For this review, take the finished solid that the model builds, in its own axes (mm). A direction names the side the tool comes from. Give positions to 0.01 mm unless a question says otherwise; leave off trailing zeros. Order: outer loops, then holes, each group sorted by start corner. A loop starts at its lowest first (then second) coordinate and runs counter-clockwise, first axis right, second up. Notation, with made-up numbers: (55, 50.5) -> (85, 50.5) arc R33 cw to (85, 86.5) -> close; hole circle Ø2 at (-9, 5). An arc over 180 degrees is marked (long way). Return JSON: item names as keys, results as strings. Group by question number.
1) Add section B-B (x = -17.8). Give the boundary of the cut face in (y, z), then the cut area to 4 significant figures.
2) Add section A-A (z = 15.5). Give the boundary of the cut face in (x, y), then the cut area to 3 significant figures.
3) Insertion check: P1, Ø2, axis at x = -17.8, z = 15.5, coming from the -Y side; P2, Ø7.5, axis at y = -9.5, z = 3, coming from the +X side; P3, Ø1.5, axis at y = -4.5, z = 9, coming from the +X side; P4, Ø8, axis at x = 10.5, y = -19.5, coming from the -Z side. Each pin has a flat end and moves straight along its axis. Give the tip position at first contact, or say it passes through.
4) For faces 1 (the face through (11.91, -15.62, 16.68)), 2 (the face through (16, -3.5, 23)), 3 (the face through (-1.05, -19, -15)), 4 (the face through (-16.9, -12.3, -14)), list the 3-axis set-ups (+Z, -Z, +X, -X, +Y, -Y) from which the entire face can be reached by the end or side of a thin tool; tool diameter is ignored.
5) Add section D-D (x = -2.3). Give the boundary of the cut face in (y, z), then the cut area to 4 significant figures.
6) To check wall thickness, follow line 1 along Z through (x, y) = (-17.8, -11.25); line 2 along X through (y, z) = (-16.25, 0); line 3 along X through (y, z) = (-19.5, -11). State the ranges of each line that lie inside material, in increasing order.
7) Add section C-C (y = -17.25). Give the boundary of the cut face in (x, z), then the cut area to 3 significant figures.
8) The part is to be moulded in two halves that separate along Z. For faces 5 (the face through (13, -3.5, 16)), 6 (the face through (16, -6.5, 23)), 7 (the face through (-21.4, -12.3, 19.2)), 8 (the face through (14.869, -4.774, -14.974)), say which applies: released by +Z, released by -Z, zero draft, split by the parting line, or undercut.
from build123d import *

# Parameters (mm, degrees)
F0_W      = 46.9
F0_H      = 42.3
F0_R      = 1.75
F1_DEPTH  = 25
F2_SIZE   = 4
F4_DEPTH  = 12.7
F5_R      = 2.1
F6_DEPTH  = 29.601
F7_SIZE   = 2
F9_DEPTH  = 25.0010001
F11_R     = 14
F12_DEPTH = 1.5


# Not quite as in the source:
# - a feature names something its author has since deleted; it is built from what else it names


with BuildPart() as f1:
    # F0 (on Front) → F1 (new body)
    with BuildSketch(Plane.XZ):
        Rectangle(F0_W, F0_H)
        with Locations((-17.8, -15.5)):
            Circle(F0_R, mode=Mode.SUBTRACT)
        with Locations((13.2, -15.5)):
            Circle(F0_R, mode=Mode.SUBTRACT)
        with Locations((-17.8, 15.5)):
            Circle(F0_R, mode=Mode.SUBTRACT)
        with Locations((13.2, 15.5)):
            Circle(F0_R, mode=Mode.SUBTRACT)
    extrude(amount=F1_DEPTH)

    # F2
    f2_edges = [f1.edges().sort_by_distance(p)[0] for p in [
        (-23.45, -12.5, 21.15),
        (23.45, -12.5, 21.15),
        (23.45, -12.5, -21.15),
        (-23.45, -12.5, -21.15),
    ]]
    chamfer(f2_edges, length=F2_SIZE)

    # F3 (on face) → F4 (cut)
    with BuildSketch(Plane(origin=(0, 0, -21.15), x_dir=(1, 0, 0), z_dir=(0, 0, -1))):
        with BuildLine():
            Line((6.95, 12.5), (14.95, 12.5))
            ThreePointArc((14.95, 12.5), (6.95, 20.5), (-1.05, 12.5))
            Line((-1.05, 12.5), (6.95, 12.5))
        make_face()
        with BuildLine():
            ThreePointArc((-1.05, 12.5), (6.95, 4.5), (14.95, 12.5))
            Line((14.95, 12.5), (6.95, 12.5))
            Line((6.95, 12.5), (-1.05, 12.5))
        make_face()
        with BuildLine():
            ThreePointArc((-1.05, 12.5), (6.95, 20.5), (14.95, 12.5))
            Line((14.95, 12.5), (14.95, 25))
            Line((14.95, 25), (-1.05, 25))
            Line((-1.05, 25), (-1.05, 12.5))
        make_face()
    extrude(amount=-F4_DEPTH, mode=Mode.SUBTRACT)

    # F5 (on face) → F6 (cut, through all)
    with BuildSketch(Plane(origin=(0, 0, -8.45), x_dir=(1, 0, 0), z_dir=(0, 0, -1))):
        with Locations((6.95, 12.5)):
            Circle(F5_R)
    extrude(amount=-F6_DEPTH, mode=Mode.SUBTRACT)

    # F7
    f7_edges = [f1.edges().sort_by_distance(p)[0] for p in [
        (4.85, -12.5, -8.45),
        (4.85, -12.5, 21.15),
    ]]
    chamfer(f7_edges, length=F7_SIZE)

    # F8 (on face) → F9 (cut, through all)
    with BuildSketch(Plane.XZ.offset(25)):
        with BuildLine():
            Line((-16.05, 15.5), (-17.8, 15.5))
            Line((-17.8, 15.5), (-16.5625631329, 14.2625631329))
            ThreePointArc((-16.5625631329, 14.2625631329), (-16.1832108181, 14.8303039934), (-16.05, 15.5))
        make_face()
        with BuildLine():
            Line((13.2, 15.5), (11.45, 15.5))
            ThreePointArc((11.45, 15.5), (11.5832108181, 14.8303039934), (11.9625631329, 14.2625631329))
            Line((11.9625631329, 14.2625631329), (13.2, 15.5))
        make_face()
        with BuildLine():
            ThreePointArc((-16.05, -15.5), (-16.1832108181, -14.8303039934), (-16.5625631329, -14.2625631329))
            Line((-16.5625631329, -14.2625631329), (-17.8, -15.5))
            Line((-17.8, -15.5), (-16.05, -15.5))
        make_face()
        with BuildLine():
            Line((3.0033008589, 5.3033008589), (-2.3, 0))
            Line((-2.3, 0), (3.0033008589, -5.3033008589))
            ThreePointArc((3.0033008589, -5.3033008589), (4.6290964938, -2.8701257427), (5.2, 0))
            ThreePointArc((5.2, 0), (4.6290964938, 2.8701257427), (3.0033008589, 5.3033008589))
        make_face()
        with BuildLine():
            ThreePointArc((3.0033008589, 5.3033008589), (-2.3, 7.5), (-7.6033008589, 5.3033008589))
            Line((-7.6033008589, 5.3033008589), (-2.3, 0))
            Line((-2.3, 0), (3.0033008589, 5.3033008589))
        make_face()
        with BuildLine():
            Line((-2.3, 0), (-7.6033008589, 5.3033008589))
            ThreePointArc((-7.6033008589, 5.3033008589), (-9.8, 0), (-7.6033008589, -5.3033008589))
            Line((-7.6033008589, -5.3033008589), (-2.3, 0))
        make_face()
        with BuildLine():
            Line((3.0033008589, -5.3033008589), (-2.3, 0))
            Line((-2.3, 0), (-7.6033008589, -5.3033008589))
            ThreePointArc((-7.6033008589, -5.3033008589), (-2.3, -7.5), (3.0033008589, -5.3033008589))
        make_face()
    extrude(amount=-F9_DEPTH, mode=Mode.SUBTRACT)

    # F11 (on offset) → F12 (join, symmetric)
    with BuildSketch(Plane.XZ.offset(5)):
        with Locations((13.2, 15.5)):
            Circle(F11_R)
    extrude(amount=F12_DEPTH, both=True)


solid = f1.part
Evaluation:
{
 "1": {"outline": "(-25, -21.15) -> (0, -21.15) -> (0, -17.25) -> (-25, -17.25) -> close; (-25, -13.75) -> (0, -13.75) -> (0, 13.75) -> (-25, 13.75) -> close; (-25, 17.25) -> (0, 17.25) -> (0, 21.15) -> (-25, 21.15) -> close", "area": "882.5 mm^2"},
 "2": {"outline": "(-23.45, -25) -> (-19.55, -25) -> (-19.55, 0) -> (-23.45, 0) -> close; (-16.05, -25) -> (11.45, -25) -> (11.45, -6.5) -> (14.95, -6.5) -> (14.95, -25) -> (23.45, -25) -> (23.45, -6.5) -> (27.2, -6.5) -> (27.2, -3.5) -> (23.45, -3.5) -> (23.45, 0) -> (14.95, 0) -> (14.95, -3.5) -> (11.45, -3.5) -> (11.45, 0) -> (-16.05, 0) -> close; hole circle Ø4.2 at (6.95, -12.5)", "area": "1,010 mm^2"},
 "3": {"P1": "through", "P2": "x = 23.45", "P3": "x = 25.96", "P4": "z = -8.45"},
 "4": {"face 1": "-Y", "face 2": "+Z, +X, +Y", "face 3": "-Z, -Y", "face 4": "+Y, -Y"},
 "5": {"outline": "(-25, -21.15) -> (0, -21.15) -> (0, -7.5) -> (-25, -7.5) -> close; (-25, 7.5) -> (0, 7.5) -> (0, 21.15) -> (-25, 21.15) -> close", "area": "682.5 mm^2"},
 "6": {"line 1": "-21.15 to -17.25, -13.75 to 13.75, 17.25 to 21.15", "line 2": "-23.45 to -9.8, 5.2 to 23.45", "line 3": "-23.45 to -1.05, 14.95 to 23.45"},
 "7": {"outline": "(-23.45, -17.15) -> (-19.45, -21.15) -> (-1.05, -21.15) -> (-1.05, -8.45) -> (14.95, -8.45) -> (14.95, -21.15) -> (19.45, -21.15) -> (23.45, -17.15) -> (23.45, 17.15) -> (19.45, 21.15) -> (-19.45, 21.15) -> (-23.45, 17.15) -> close; hole circle Ø3.5 at (-17.8, -15.5); hole circle Ø3.5 at (-17.8, 15.5); hole circle Ø15 at (-2.3, 0); hole circle Ø3.5 at (13.2, 15.5)", "area": "1,540 mm^2"},
 "8": {"face 5": "undercut", "face 6": "zero draft", "face 7": "released by +Z", "face 8": "undercut"}
}
